```python
from build123d import *

# Parameters (mm, degrees)
F0_W       = 34.5
F0_H       = 18.5
F1_DEPTH   = 28
F2_R       = 2
F3_DEPTH   = 19
F4_SIZE    = 8
F5_SIZE2   = 8
F5_SIZE    = 25
F5_2_SIZE2 = 8
F5_2_SIZE  = 25
F6_SIZE2   = 2
F6_SIZE    = 25
F6_2_SIZE2 = 2
F6_2_SIZE  = 25
F7_R       = 2
F8_R       = 2.8


with BuildPart() as f1:
    # F0 (on Front) → F1 (new body)
    with BuildSketch(Plane.XZ):
        Rectangle(F0_W, F0_H)
    extrude(amount=-F1_DEPTH)

    # F2 (on face) → F3 (join)
    with BuildSketch(Plane.XZ):
        with Locations((-8.5, -2)):
            Circle(F2_R)
        with Locations((8.5, -2)):
            Circle(F2_R)
        with Locations((0, 3)):
            Circle(F2_R)
    extrude(amount=F3_DEPTH)

    # F4
    f4_edges = [f1.edges().sort_by_distance(p)[0] for p in [
        (17.25, 14, 9.25),
        (-17.25, 14, 9.25),
        (17.25, 14, -9.25),
        (-17.25, 14, -9.25),
    ]]
    chamfer(f4_edges, length=F4_SIZE)

    # F5
    f5_edges = [f1.edges().sort_by_distance(p)[0] for p in [
        (17.25, 28, 0),
    ]]
    f5_side = f1.faces().sort_by_distance((17.25, 14, 0))[0]
    chamfer(f5_edges, length=F5_SIZE, length2=F5_SIZE2, reference=f5_side)

    # F5#2
    f5_2_edges = [f1.edges().sort_by_distance(p)[0] for p in [
        (-17.25, 28, 0),
    ]]
    f5_2_side = f1.faces().sort_by_distance((-17.25, 14, 0))[0]
    chamfer(f5_2_edges, length=F5_2_SIZE, length2=F5_2_SIZE2, reference=f5_2_side)

    # F6
    f6_edges = [f1.edges().sort_by_distance(p)[0] for p in [
        (0, 28, 9.25),
    ]]
    f6_side = f1.faces().sort_by_distance((0, 14, 9.25))[0]
    chamfer(f6_edges, length=F6_SIZE, length2=F6_SIZE2, reference=f6_side)

    # F6#2
    f6_2_edges = [f1.edges().sort_by_distance(p)[0] for p in [
        (0, 28, -9.25),
    ]]
    f6_2_side = f1.faces().sort_by_distance((0, 14, -9.25))[0]
    chamfer(f6_2_edges, length=F6_2_SIZE, length2=F6_2_SIZE2, reference=f6_2_side)

    # F7
    f7_edges = [f1.edges().sort_by_distance(p)[0] for p in [
        (-10.5, -19, -2),
        (6.5, -19, -2),
        (-2, -19, 3),
    ]]
    fillet(f7_edges, radius=F7_R)

    # F8
    f8_edges = [f1.edges().sort_by_distance(p)[0] for p in [
        (-17.25, 1.5, 1.25),
        (-17.25, 1.5, -1.25),
        (17.25, 1.5, 1.25),
        (17.25, 1.5, -1.25),
    ]]
    fillet(f8_edges, radius=F8_R)


solid = f1.part
```
Here's how the part is built. I have some questions about the finished solid (model axes, mm). A direction names the side the tool comes from. Give positions to 0.01 mm unless a question says otherwise; leave off trailing zeros. Loops run counter-clockwise (first coordinate to the right, second up) from the corner with the lowest first, then second, coordinate; pieces in that order, holes last. Notation, with made-up numbers: (-28.5, 18) -> (24.5, 18) arc R28 ccw to (24.5, 40) -> close; hole circle Ø8 at (-16, 17). An arc over 180 degrees is marked (long way). Use one line per item in the form item = value. Start each with the question number.
1) Thinking about a two-plate mould opening in X: for faces 1 (the face through (16.926, 2.202, 1.397)), 2 (the face through (-12.8, 8.8, 5.7)), 3 (the face through (6.502, -8.381, -1.912)), which applies, +X half, -X half, draft (parallel to the pull), parting line (faces both ways), or undercut?
2) Imagine slicing it at C-C (y = 8). Please give me the cut outline in (x, z), then the cut area to 3 significant figures.
3) Imagine slicing it at D-D (z = 3). Please give me the cut outline in (x, y), then the cut area to 3 significant figures.
4) Imagine slicing it at B-B (x = 8.5). Please give me the cut outline in (y, z), then the cut area to 3 significant figures.
5) Which directions (+Z, -Z, +X, -X, +Y, -Y) give clear straight access to the entire face, cutting with the end or side of a thin tool? Please do faces 4 (the face through (0, 0, 0)), 5 (the face through (-17.04, 2.2, 1.15)).
6) Please list where these lines run through material, in increasing order: line 1 along Y through (x, z) = (5, 5.25); line 2 along X through (y, z) = (-17, -3); line 3 along X through (y, z) = (-7, -2.5).
7) Imagine slicing it at A-A (y = -15). Please give me the cut outline in (x, z).
8) For P1, Ø5, axis at y = 19.5, z = 1.5, coming from the -X side; P2, Ø6, axis at x = 6.5, y = 14.5, coming from the -Z side; P3, Ø3, axis at x = 2, y = 7.5, coming from the +Z side, each with a flat end and sliding along its axis, tell me the tip position at first contact or that it passes through.
Check values:
q1.face_1 = +X half
q1.face_2 = -X half
q1.face_3 = undercut
q2.outline = (-15.65, -2.85) -> (-9.65, -8.85) -> (9.65, -8.85) -> (15.65, -2.85) -> (15.65, 2.85) -> (9.65, 8.85) -> (-9.65, 8.85) -> (-15.65, 2.85) -> close
q2.area = 482 mm^2
q3.outline = (-15.5, 0) -> (-2, 0) -> (-2, -17) arc R2 ccw to (2, -17) -> (2, 0) -> (15.5, 0) -> (15.5, 8.47) -> (9.25, 28) -> (-9.25, 28) -> (-15.5, 8.47) -> close
q3.area = 820 mm^2
q4.outline = (-17, -4) -> (0, -4) -> (0, -9.25) -> (3, -9.25) -> (28, -7.25) -> (28, 7.25) -> (3, 9.25) -> (0, 9.25) -> (0, 0) -> (-17, 0) arc R2 ccw to start
q4.area = 542 mm^2
q5.face_4 = -Y
q5.face_5 = +Z, -X, +Y, -Y
q6.line_1 = 0 to 28
q6.line_2 = -10.23 to -6.77, 6.77 to 10.23
q6.line_3 = -10.44 to -6.56, 6.56 to 10.44
q7.outline = circle Ø4 at (-8.5, -2); circle Ø4 at (0, 3); circle Ø4 at (8.5, -2)
q8.P1 = -12.77
q8.P2 = -8.57
q8.P3 = 9.01
